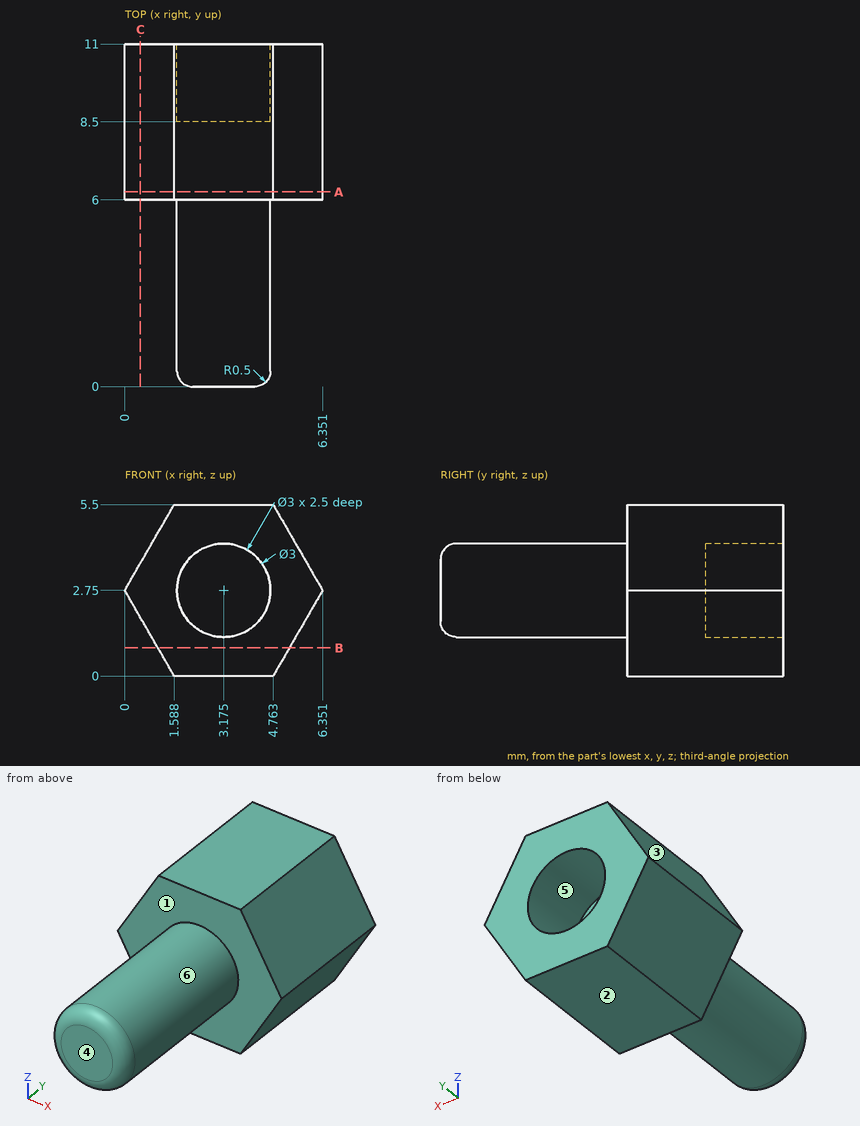
Job drawing, mm, ordinate dimensions from the low corner. One solid piece. A direction names the side the tool comes from. Give positions to 0.01 mm unless a question says otherwise; leave off trailing zeros. Loops run counter-clockwise (first coordinate to the right, second up) from the corner with the lowest first, then second, coordinate; pieces in that order, holes last. Notation, with made-up numbers: M -22.5,-36.5 L 14.5,-36.5 A19 ccw 14.5,-17.5 Z; hole C 21.25,58 d6. An arc over 180 degrees is marked long. Put each result on its own line as item: value. Start each with the question number.
1) Pull direction X, two halves, no side cores. Call the marked faces 3, 4, 5 and 6: +X half, -X half, draft (parallel to the pull), parting line (faces both ways), or undercut.
2) Saw through at C-C (x = 0.5). List the corners of the cut face in (y, z).
3) Saw through at A-A (y = 6.25). List the corners of the cut face in (x, z), then the cut area to 3 significant figures.
4) Probe probe 1 along Y at (x, z) = (3.25, 4.4); probe 2 along Z at (x, y) = (2.25, 10.75); probe 3 along Y at (x, z) = (3.25, 1.5). List the from-to ranges inside material, lowest first.
5) Saw through at B-B (z = 0.9). List the corners of the cut face in (x, y), then the cut area to 3 significant figures.
6) 3-axis set-ups, long thin cutter, end or side, ignore diameter. For the marked faces 1 and 2: which of +Z, -Z, +X, -X, +Y, -Y reach the whole face in a straight line?
Numbers:
1. face 3: -X half
1. face 4: draft
1. face 5: undercut
1. face 6: parting line
2. outline: M 6,1.88 L 11,1.88 L 11,3.62 L 6,3.62 Z
3. outline: M 0,2.75 L 1.59,0 L 4.76,0 L 6.35,2.75 L 4.76,5.5 L 1.59,5.5 Z
3. area: 26.2 mm^2
4. probe 1: 6 to 11
4. probe 2: 0 to 1.57, 3.93 to 5.5
4. probe 3: 0.07 to 8.5
5. outline: M 1.07,6 L 5.28,6 L 5.28,11 L 1.07,11 Z
5. area: 21.1 mm^2
6. face 1: -Y
6. face 2: -Z, +X, -X, +Y, -Y
